Geometry: final body of the model. Coordinates: model frame, mm. Face numbers are marked on the shaded views. A direction names the side the tool comes from. Give positions to 0.01 mm unless a question says otherwise; leave off trailing zeros. Write each loop counter-clockwise with the first axis right and the second up, starting at its lowest first coordinate (ties: lowest second). Pieces come first, ordered by that corner, then holes. Notation, with made-up numbers: (-26.5, 44.5) -> (0.5, 44.5) arc R21 cw to (0.5, 67.5) -> close; hole circle Ø6 at (26, 50.25). An arc over 180 degrees is marked (long way). Answer in a Markdown table with one row per item. Add a question column.
from build123d import *

# Parameters (mm, degrees)
F0_W     = 48.783202
F0_H     = 6.73111
F1_DEPTH = 3.302
F2_R     = 1.6
F3_DEPTH = 32


with BuildPart() as f1:
    # F0 (on Front) → F1 (new body)
    with BuildSketch(Plane.XZ):
        with Locations((24.391601, 3.365555)):
            Rectangle(F0_W, F0_H)
    extrude(amount=-F1_DEPTH)

    # F2 (on Top) → F3 (join)
    with BuildSketch(Plane.XY):
        with Locations((3.1, 1.626936)):
            Circle(F2_R)
        with Locations((7.799981, 1.640332)):
            Circle(F2_R)
        with Locations((12.369818, 1.623737)):
            Circle(F2_R)
        with Locations((36.283233, 1.66498)):
            Circle(F2_R)
        with Locations((40.983233, 1.66498)):
            Circle(F2_R)
        with Locations((45.683233, 1.66498)):
            Circle(F2_R)
    extrude(amount=F3_DEPTH)


solid = f1.part
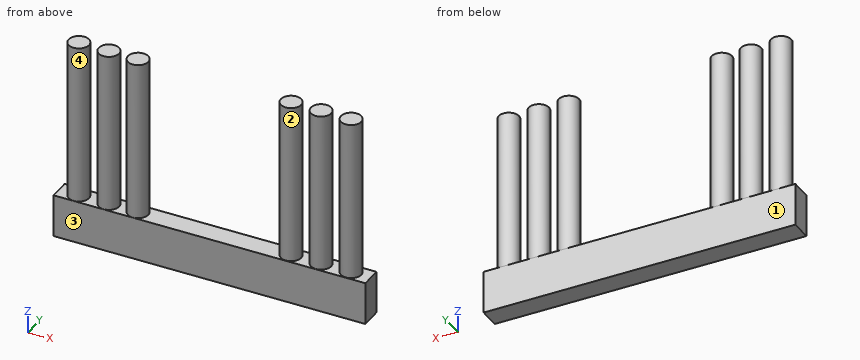
Q1. Section D-D on x = 35.5. Return loops of the section in (y, z), and give its area (3 significant figures).
Q2. Access query for the marked faces 3 and 4. Directions: +Z, -Z, +X, -X, +Y, -Y. A direction counts if a zero-diameter tool reaches every point of the face in a straight line with its end or side. Return the directions, or none.
Q3. Section A-A on z = 21. Return loops of the section in (x, y).
Q4. Contact query for flat-ended pins moving along their axis: pin 1 Ø1 at (x, y) = (25, 2.5) entering from +Z; pin 2 Ø1.5 at (y, z) = (0.5, 18) entering from -X; pin 3 Ø1 at (y, z) = (3, 9) entering from +X. Output: stop coordinate, or through.
Q5. Section B-B on y = 0.8. Return loops of the section in (x, z).
Q6. Pull-direction query (X, two-part tool) for the marked faces 1 and 2; classes: +X half, -X half, draft (parallel to the pull), parting line (faces both ways), or undercut.
Q7. Line query: probe 1 along X at (y, z) = (1.65, 26); probe 2 along X at (y, z) = (2.4, 19); probe 3 along Z at (x, y) = (14, 2.45). Output: solid intervals per line, ascending. Write a range as from..to.
Checks:
| question | item | result |
|---|---|---|
| 1 | outline | (0, 0) -> (3.3, 0) -> (3.3, 6.73) -> (3.06, 6.73) -> (3.06, 32) -> (0.27, 32) -> (0.27, 6.73) -> (0, 6.73) -> close |
| 1 | area | 92.7 mm^2 |
| 2 | face 3 | +Z, -Z, +X, -X, -Y |
| 2 | face 4 | +Z |
| 3 | outline | circle Ø3.2 at (3.1, 1.63); circle Ø3.2 at (7.8, 1.64); circle Ø3.2 at (12.37, 1.62); circle Ø3.2 at (36.28, 1.66); circle Ø3.2 at (40.98, 1.66); circle Ø3.2 at (45.68, 1.66) |
| 4 | pin 1 | z = 6.73 |
| 4 | pin 2 | x = 1.55 |
| 4 | pin 3 | x = 47.05 |
| 5 | outline | (0, 0) -> (48.78, 0) -> (48.78, 6.73) -> (47.03, 6.73) -> (47.03, 32) -> (44.34, 32) -> (44.34, 6.73) -> (42.33, 6.73) -> (42.33, 32) -> (39.64, 32) -> (39.64, 6.73) -> (37.63, 6.73) -> (37.63, 32) -> (34.94, 32) -> (34.94, 6.73) -> (13.74, 6.73) -> (13.74, 32) -> (11, 32) -> (11, 6.73) -> (9.16, 6.73) -> (9.16, 32) -> (6.44, 32) -> (6.44, 6.73) -> (4.47, 6.73) -> (4.47, 32) -> (1.73, 32) -> (1.73, 6.73) -> (0, 6.73) -> close |
| 6 | face 1 | draft |
| 6 | face 2 | undercut |
| 7 | probe 1 | 1.5..4.7, 6.2..9.4, 10.77..13.97, 34.68..37.88, 39.38..42.58, 44.08..47.28 |
| 7 | probe 2 | 1.7..4.5, 6.39..9.21, 10.97..13.77, 34.86..37.7, 39.56..42.4, 44.26..47.1 |
| 7 | probe 3 | 0..6.73 |
